The model under review builds one solid part; all positions refer to its coordinate system, in mm. Face numbers are marked on the shaded views. A direction names the side the tool comes from. Coordinates: 2 decimals unless noted, no trailing zeros. Order: outer loops, then holes, each group sorted by start corner. A loop starts at its lowest first (then second) coordinate and runs counter-clockwise, first axis right, second up. Notation, with made-up numbers: (37, 11) - (59, 11) arc R20 ccw to (59, 37) - close; hole circle Ø1 at (54.5, 86.25). An arc over 180 degrees is marked (long way). Answer in a Markdown table with one row per item.
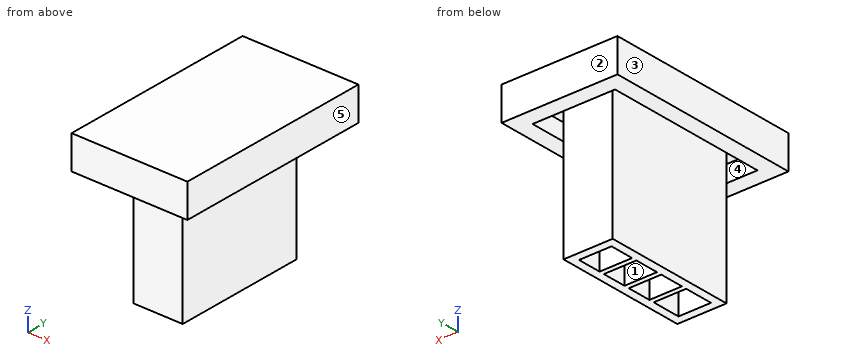
```python
from build123d import *

# Parameters (mm, degrees)
SKETCH1_W           = 2.95
SKETCH1_H           = 7.95
BOSS_EXTRUDE1_DEPTH = 8
SHELL1_T            = -0.5
SKETCH2_W           = 4.95
SKETCH2_H           = 9.95
BOSS_EXTRUDE2_DEPTH = 1
SKETCH3_W           = 1.95
SKETCH3_H           = 0.3
BOSS_EXTRUDE3_DEPTH = 7.5
SKETCH4_W           = 6.95
SKETCH4_H           = 11.95
SKETCH4_W_2         = 4.95
SKETCH4_H_2         = 9.95
BOSS_EXTRUDE5_DEPTH = 2


with BuildPart() as part:
    # Sketch1 → Boss-Extrude1 (new body)
    with BuildSketch(Plane.XY):
        with Locations((0.443379447, -2.741798419)):
            Rectangle(SKETCH1_W, SKETCH1_H)
    extrude(amount=BOSS_EXTRUDE1_DEPTH)

    # Shell1
    shell1_openings = [part.faces().sort_by_distance(p)[0] for p in [
        (0.443379447, -2.741798419, 0),
    ]]
    offset(amount=SHELL1_T, openings=shell1_openings, kind=Kind.INTERSECTION)

    # Sketch2 → Boss-Extrude2 (add)
    with BuildSketch(Plane.XY.offset(8)):
        with Locations((0.443379447, -2.741798419)):
            Rectangle(SKETCH2_W, SKETCH2_H)
    extrude(amount=BOSS_EXTRUDE2_DEPTH)

    # Sketch3 → Boss-Extrude3 (add)
    with BuildSketch(Plane(origin=(0, 0, 7.5), x_dir=(-1, 0, 0), z_dir=(0, 0, -1))):
        with Locations((-0.443379447, -0.854298419)):
            Rectangle(SKETCH3_W, SKETCH3_H)
        with Locations((-0.443379447, -2.594298419)):
            Rectangle(SKETCH3_W, SKETCH3_H)
        with Locations((-0.443379447, -4.334298419)):
            Rectangle(SKETCH3_W, SKETCH3_H)
    extrude(amount=BOSS_EXTRUDE3_DEPTH)

    # Sketch4 → Boss-Extrude5 (add)
    with BuildSketch(Plane.XY.offset(9)):
        with Locations((0.443379447, -2.741798419)):
            Rectangle(SKETCH4_W, SKETCH4_H)
        with Locations((0.443379447, -2.741798419)):
            Rectangle(SKETCH4_W_2, SKETCH4_H_2, mode=Mode.SUBTRACT)
    extrude(amount=-BOSS_EXTRUDE5_DEPTH)


solid = part.part
```
Item 1: To check wall thickness, follow line 1 (Y direction, x = 0, z = 5.75); line 2 (X direction, y = -3.5, z = 5); line 3 (Z direction, x = 3.5, y = -2.25). State the ranges of each line that lie inside material, in increasing order. Write a range as from..to.
Check values:
| item | result |
|---|---|
| line 1 | -6.72..-6.22, -4.48..-4.18, -2.74..-2.44, -1..-0.7, 0.73..1.23 |
| line 2 | -1.03..-0.53, 1.42..1.92 |
| line 3 | 7..9 |
Item 2: We need section A-A, the plane z = 7.75. Write out the cut boundary in (x, y).
Check values:
| item | result |
|---|---|
| outline | (-3.03, -8.72) - (3.92, -8.72) - (3.92, 3.23) - (-3.03, 3.23) - close; (-1.03, -6.72) - (1.92, -6.72) - (1.92, 1.23) - (-1.03, 1.23) - close; hole (-2.03, -7.72) - (2.92, -7.72) - (2.92, 2.23) - (-2.03, 2.23) - close |
Item 3: We need section B-B, the plane x = 2.25. Write out the cut boundary in (y, z).
Check values:
| item | result |
|---|---|
| outline | (-8.72, 7) - (-7.72, 7) - (-7.72, 8) - (2.23, 8) - (2.23, 7) - (3.23, 7) - (3.23, 9) - (-8.72, 9) - close |
Item 4: We need section D-D, the plane z = 2.5. Write out the cut boundary in (x, y).
Check values:
| item | result |
|---|---|
| outline | (-1.03, -6.72) - (1.92, -6.72) - (1.92, 1.23) - (-1.03, 1.23) - close; hole (-0.53, -6.22) - (1.42, -6.22) - (1.42, -4.48) - (-0.53, -4.48) - close; hole (-0.53, -4.18) - (1.42, -4.18) - (1.42, -2.74) - (-0.53, -2.74) - close; hole (-0.53, -2.44) - (1.42, -2.44) - (1.42, -1) - (-0.53, -1) - close; hole (-0.53, -0.7) - (1.42, -0.7) - (1.42, 0.73) - (-0.53, 0.73) - close |
Item 5: Clearance check with flat-ended pins moving along their axes: pin 1 Ø1.6 at (y, z) = (-3.5, 2.5) entering from +X; pin 2 Ø3 at (x, z) = (-1.5, 2) entering from +Y; pin 3 Ø1.6 at (y, z) = (-1.5, 3) entering from -X; pin 4 Ø1.2 at (x, y) = (0, -1.5) entering from -Z. State where each tip first meets the part, or that it passes through.
Check values:
| item | result |
|---|---|
| pin 1 | x = 1.92 |
| pin 2 | y = 1.23 |
| pin 3 | x = -1.03 |
| pin 4 | z = 0 |
Item 6: We need section C-C, the plane y = 1.5. Write out the cut boundary in (x, z).
Check values:
| item | result |
|---|---|
| outline | (-3.03, 7) - (-2.03, 7) - (-2.03, 8) - (2.92, 8) - (2.92, 7) - (3.92, 7) - (3.92, 9) - (-3.03, 9) - close |
Item 7: Tool access review of the marked faces 4 and 5: name each direction out of +Z, -Z, +X, -X, +Y, -Y from which nothing blocks a thin tool from reaching the whole face with its end or side.
Check values:
| item | result |
|---|---|
| face 4 | -Z |
| face 5 | +Z, -Z, +X, +Y, -Y |
Item 8: Mouldability with a two-part tool opening along Y and no side actions: class the marked faces 1, 2 and 3 as +Y half, -Y half, draft (parallel to the pull), parting line (faces both ways), or undercut.
Check values:
| item | result |
|---|---|
| face 1 | undercut |
| face 2 | +Y half |
| face 3 | draft |
